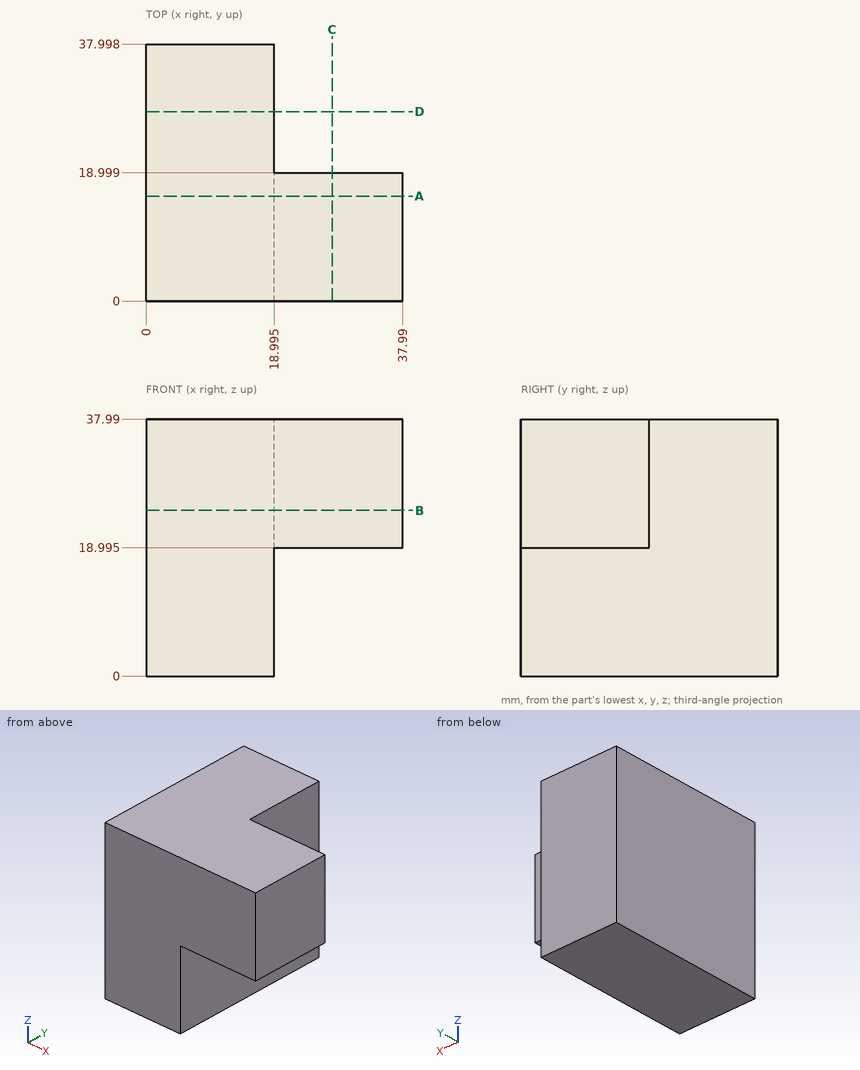
Part print with two shaded views. Sizes in mm from the minimum x, y, z corner. Give positions to 0.01 mm unless a question says otherwise; leave off trailing zeros. Write each loop counter-clockwise with the first axis right and the second up, starting at its lowest first coordinate (ties: lowest second). Pieces come first, ordered by that corner, then holes.
1) Cut at B-B on z = 24.5. Write the cut outline in (x, y) (1 decimal), then the cut area to 3 significant figures.
Resolved:
outline: (0, 0) - (38, 0) - (38, 19) - (19, 19) - (19, 38) - (0, 38) - close
area: 1,080 mm2
2) Cut at D-D on y = 28. Write the cut outline in (x, z) (1 decimal).
Resolved:
outline: (0, 0) - (19, 0) - (19, 38) - (0, 38) - close
3) Cut at A-A on y = 15.5. Write the cut outline in (x, z) (1 decimal), then the cut area to 3 significant figures.
Resolved:
outline: (0, 0) - (19, 0) - (19, 19) - (38, 19) - (38, 38) - (0, 38) - close
area: 1,080 mm2
4) Pin check, flat tips, straight feed: pin 1 (15 mm diameter, centred on x = 25.5, z = 27, fed in from +Y); pin 2 (5 mm diameter, centred on y = 27.5, z = 7, fed in from +X) (1 decimal). Stop position of each tip, or through.
Resolved:
pin 1: stops at y = 38
pin 2: stops at x = 19
5) Cut at C-C on x = 27.5. Write the cut outline in (y, z) (1 decimal).
Resolved:
outline: (0, 19) - (19, 19) - (19, 38) - (0, 38) - close
6) Probe L1, parallel to X at y = 4, z = 4 (1 decimal); L2, parallel to Z at x = 33.5, y = 16.5 (1 decimal). List the from-to ranges inside material, lowest first.
Resolved:
L1: x = 0 to 19
L2: z = 19 to 38
